from build123d import *

# Parameters (mm, degrees)
CROQUIS1_W              = 47
CROQUIS1_H              = 34.25
SALIENTE_EXTRUIR1_DEPTH = 1.5
CROQUIS2_W              = 9
CROQUIS2_H              = 12.2
CORTAR_EXTRUIR5_DEPTH   = 21.5
CORTAR_EXTRUIR6_DEPTH   = 21.5


with BuildPart() as part:
    # Croquis1 → Saliente-Extruir1 (new body)
    with BuildSketch(Plane.XY):
        with Locations((-1.565239082, -10.286716172)):
            Rectangle(CROQUIS1_W, CROQUIS1_H)
    extrude(amount=SALIENTE_EXTRUIR1_DEPTH)

    # Croquis2 → Cortar-Extruir5 (cut)
    with BuildSketch(Plane.XY):
        with Locations((-6.065239082, -6.761716172)):
            Rectangle(CROQUIS2_W, CROQUIS2_H)
    extrude(amount=CORTAR_EXTRUIR5_DEPTH, mode=Mode.SUBTRACT)

    # Croquis3 → Cortar-Extruir6 (cut)
    with BuildSketch(Plane.XY):
        with BuildLine():
            Line((-25.065239082, -25.911716172), (-25.065239082, -27.411716172))
            Line((-25.065239082, -27.411716172), (-23.565239082, -27.411716172))
            ThreePointArc((-23.565239082, -27.411716172), (-24.625899254, -26.972376343), (-25.065239082, -25.911716172))
        make_face()
        with BuildLine():
            Line((-25.065239082, 5.338283828), (-25.065239082, 6.838283828))
            Line((-25.065239082, 6.838283828), (-23.565239082, 6.838283828))
            ThreePointArc((-23.565239082, 6.838283828), (-24.625899254, 6.398944), (-25.065239082, 5.338283828))
        make_face()
        with BuildLine():
            Line((20.434760918, 6.838283828), (21.934760918, 6.838283828))
            Line((21.934760918, 6.838283828), (21.934760918, 5.338283828))
            ThreePointArc((21.934760918, 5.338283828), (21.49542109, 6.398944), (20.434760918, 6.838283828))
        make_face()
        with BuildLine():
            Line((21.934760918, -27.411716172), (21.934760918, -25.911716172))
            ThreePointArc((21.934760918, -25.911716172), (21.49542109, -26.972376343), (20.434760918, -27.411716172))
            Line((20.434760918, -27.411716172), (21.934760918, -27.411716172))
        make_face()
    extrude(amount=CORTAR_EXTRUIR6_DEPTH, mode=Mode.SUBTRACT)


solid = part.part
Work out the finished part from the listing and answer in its coordinate system (mm). A direction names the side the tool comes from. Coordinates: 2 decimals unless noted, no trailing zeros. Write each loop counter-clockwise with the first axis right and the second up, starting at its lowest first coordinate (ties: lowest second). Pieces come first, ordered by that corner, then holes. Notation, with made-up numbers: M -12,82 L 42,82 A30 ccw 42,110 Z; hole C -36.5,76.5 d2. An arc over 180 degrees is marked long. Write item = value, one per line.
1. For faces 4 (the face through (-1.565, -7, 1)), 5 (the face through (-2, -14, 1.5)), determine the directions among +Z, -Z, +X, -X, +Y, -Y from which every point of the face is accessible in a straight line to the end or side of a thin tool.
Solution:
face_4 = +Z, -Z
face_5 = +Z, +X, -X, +Y, -Y
2. Determine the mould class of faces 1 (the face through (-2, -14, 0)), 2 (the face through (-24.614, 6.411, 0.74)), 3 (the face through (-10.565, -7, 1)) for opening direction Y: released by +Y, released by -Y, zero draft, split by the parting line, or undercut.
Solution:
face_1 = zero draft
face_2 = released by +Y
face_3 = undercut
3. The part is cut by section B-B (y = -2). Determine the outline of the cut face in (x, z), then the cut area to 3 significant figures.
Solution:
outline = M -25.07,0 L -10.57,0 L -10.57,1.5 L -25.07,1.5 Z; M -1.57,0 L 21.93,0 L 21.93,1.5 L -1.57,1.5 Z
area = 57.0 mm2
4. The part is cut by section A-A (x = -4). Determine the outline of the cut face in (y, z), then the cut area to 3 significant figures.
Solution:
outline = M -27.41,0 L -12.86,0 L -12.86,1.5 L -27.41,1.5 Z; M -0.66,0 L 6.84,0 L 6.84,1.5 L -0.66,1.5 Z
area = 33.1 mm2
5. Straight lines are drawn through the part: line 1 (X direction, y = -10, z = 0.3); line 2 (Y direction, x = -2, z = 0.65). For each, find the intervals that lie inside material, in ascending order. Write a range as from..to.
Solution:
line_1 = -25.07..-10.57, -1.57..21.93
line_2 = -27.41..-12.86, -0.66..6.84
6. The part is cut by section C-C (z = 1.25). Determine the outline of the cut face in (x, y).
Solution:
outline = M -25.07,-25.91 A1.5 ccw -23.57,-27.41 L 20.43,-27.41 A1.5 ccw 21.93,-25.91 L 21.93,5.34 A1.5 ccw 20.43,6.84 L -23.57,6.84 A1.5 ccw -25.07,5.34 Z; hole M -10.57,-12.86 L -1.57,-12.86 L -1.57,-0.66 L -10.57,-0.66 Z
